Source: CAD feature listing. Evaluate the final solid. Frame: model axes, mm. A direction names the side the tool comes from. Round coordinates to 2 decimals unless told otherwise and drop trailing zeros. Order: outer loops, then holes, each group sorted by start corner. A loop starts at its lowest first (then second) coordinate and runs counter-clockwise, first axis right, second up. Notation, with made-up numbers: (65, 16) -> (116, 16) arc R33 cw to (116, 53) -> close; hole circle Ø2 at (43.5, -14.75). An arc over 180 degrees is marked (long way). One line per item, written item: value. Start each with the question number.
1) Ray query, L1, parallel to Z at x = 11.75, y = 0.25; L2, parallel to X at y = 1.4, z = 14.5; L3, parallel to X at y = 0.6, z = -21.5. Return the intervals inside material, ascending.
2) Pin query (flat end, axial travel): P1, Ø0.8, axis at y = 0.5, z = 19.5, coming from the -X side; P2, Ø0.5, axis at x = 11.5, y = 1, coming from the -Z side. Return the tip coordinate at first contact, or that it passes through.
3) Section A-A (z = 25). Return the cut outline in (x, y), and give its area (3 significant figures).
4) Reachability of faces 1 (the face through (11.112, 1, -18)), 2 (the face through (-12, 1, -7.938)), 3 (the face through (-12, 1, 11.112)), 4 (the face through (-3, 0, 6)), 5 (the face through (12, 1, 11.112)) from +Z, -Z, +X, -X, +Y, -Y: full face, straight path, thin tool, end or side. Return the list, or none.
```python
from build123d import *

# Parameters (mm, degrees)
SKETCH1_W           = 1.5875
SKETCH1_H           = 19.05
BOSS_EXTRUDE1_DEPTH = 1.5875


with BuildPart() as part:
    # Sketch1 → Boss-Extrude1 (new body)
    with BuildSketch(Plane(origin=(0, 0, 0), x_dir=(1, 0, 0), z_dir=(0, 1, 0))):
        with BuildLine():
            Line((11.1125, 7.9375), (11.1125, 29.02868761))
            add(Edge.make_bspline(
                [(-11.1125, 29.02868761), (0, -16.161766196), (11.1125, 29.02868761)],
                knots=[2.076156837, 2.076156837, 2.076156837, 4.20702847, 4.20702847, 4.20702847], degree=2, weights=[1, 0.484122918, 1]))
            Line((-11.1125, 29.02868761), (-11.1125, 7.9375))
            Line((-11.1125, 7.9375), (-11.1125, -11.1125))
            Line((-11.1125, -11.1125), (-11.1125, -42.8625))
            ThreePointArc((-11.1125, -42.8625), (0, -31.75), (11.1125, -42.8625))
            Line((11.1125, -42.8625), (11.1125, -11.1125))
            Line((11.1125, -11.1125), (11.1125, 7.9375))
        make_face()
        with Locations((11.90625, -1.5875)):
            Rectangle(SKETCH1_W, SKETCH1_H)
        with Locations((-11.90625, -1.5875)):
            Rectangle(SKETCH1_W, SKETCH1_H)
    extrude(amount=BOSS_EXTRUDE1_DEPTH)


solid = part.part
```
Findings:
1. L1: -7.94 to 11.11
1. L2: -11.11 to 11.11
1. L3: -11.11 to -8.43, 8.43 to 11.11
2. P1: x = -11.11
2. P2: z = -7.94
3. outline: (-11.11, 0) -> (11.11, 0) -> (11.11, 1.59) -> (-11.11, 1.59) -> close
3. area: 35.3 mm2
4. face 1: -Z, +X, +Y, -Y
4. face 2: -Z, -X, +Y, -Y
4. face 3: +Z, -X, +Y, -Y
4. face 4: +Z, -Z, +X, -X, -Y
4. face 5: +Z, +X, +Y, -Y
